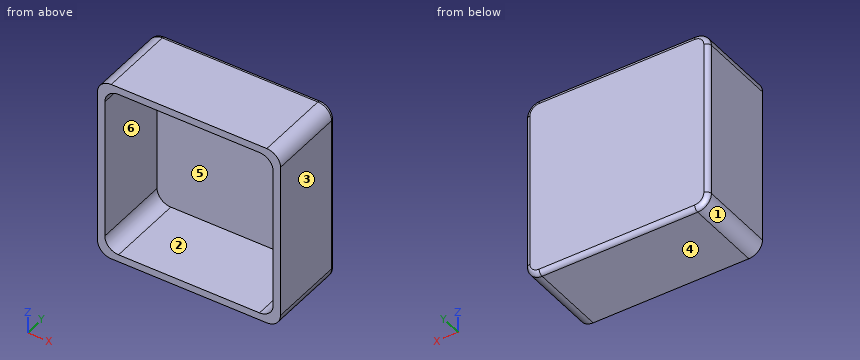
from build123d import *

# Parameters (mm, degrees)
F0_W     = 200
F0_H     = 200
F0_W_2   = 184
F0_H_2   = 184
F1_DEPTH = 85
F2_R     = 15
F4_DEPTH = 3
F5_R     = 5


with BuildPart() as f1:
    # F0 (on Front) → F1 (new body)
    with BuildSketch(Plane.XZ):
        Rectangle(F0_W, F0_H)
        Rectangle(F0_W_2, F0_H_2, mode=Mode.SUBTRACT)
    extrude(amount=F1_DEPTH)

    # F2
    f2_edges = [f1.edges().sort_by_distance(p)[0] for p in [
        (-100, -42.5, 100),
        (-92, -42.5, 92),
        (100, -42.5, 100),
        (92, -42.5, 92),
        (100, -42.5, -100),
        (92, -42.5, -92),
        (-92, -42.5, -92),
        (-100, -42.5, -100),
    ]]
    fillet(f2_edges, radius=F2_R)

    # F3 (on face) → F4 (join)
    with BuildSketch(Plane(origin=(0, 0, 0), x_dir=(-1, 0, 0), z_dir=(0, 1, 0))):
        with BuildLine():
            Line((-85, -100), (85, -100))
            ThreePointArc((85, -100), (95.606602, -95.606602), (100, -85))
            Line((100, -85), (100, 85))
            ThreePointArc((100, 85), (95.606602, 95.606602), (85, 100))
            Line((85, 100), (-85, 100))
            ThreePointArc((-85, 100), (-95.606602, 95.606602), (-100, 85))
            Line((-100, 85), (-100, -85))
            ThreePointArc((-100, -85), (-95.606602, -95.606602), (-85, -100))
        make_face()
    extrude(amount=F4_DEPTH)

    # F5
    f5_edges = [f1.edges().sort_by_distance(p)[0] for p in [
        (95.606602, 3, -95.606602),
    ]]
    fillet(f5_edges, radius=F5_R)


solid = f1.part
The listing builds one solid part. Answer for the finished solid, in the listing's coordinates (mm). Face numbers are marked on the shaded views. A direction names the side the tool comes from. Give positions to 0.01 mm unless a question says otherwise; leave off trailing zeros. Order: outer loops, then holes, each group sorted by start corner. A loop starts at its lowest first (then second) coordinate and runs counter-clockwise, first axis right, second up. Notation, with made-up numbers: (-16.5, 60) - (42.5, 60) arc R7 ccw to (42.5, 67) - close; hole circle Ø7 at (-29.5, 70). An arc over 180 degrees is marked (long way). Answer as CSV lines item,"result".
Q1. Determine the mould class of the marked faces 3, 4, 5 and 6 for opening direction X: pulls with the +X half, pulls with the -X half, needs draft (parallel to the pull), parting line crosses it, or undercut.
Answer key:
face 3,"pulls with the +X half"
face 4,"needs draft"
face 5,"undercut"
face 6,"undercut"
Q2. A cutting plane is placed at C-C, the plane x = 15. Determine the outline of the cut face in (y, z).
Answer key:
outline,"(-85, -100) - (-2, -100) arc R5 ccw to (3, -95) - (3, 95) arc R5 ccw to (-2, 100) - (-85, 100) - (-85, 92) - (0, 92) - (0, -92) - (-85, -92) - close"
Q3. Which of the six approach directions +Z, -Z, +X, -X, +Y, -Y give full straight-line access (tool end or side, diameter ignored) to the marked faces 1 and 2?
Answer key:
face 1,"-Z, -X, +Y, -Y"
face 2,"-Y"
Q4. Straight lines are drawn through the part: L1, parallel to Z at x = -67.5, y = -15; L2, parallel to Y at x = 11, z = -60. For each, find the intervals that lie inside material, in ascending order.
Answer key:
L1,"z = -100 to -92, 92 to 100"
L2,"y = 0 to 3"
Q5. A cutting plane is placed at A-A, the plane y = -15. Determine the outline of the cut face in (x, z).
Answer key:
outline,"(-100, -85) arc R15 ccw to (-85, -100) - (85, -100) arc R15 ccw to (100, -85) - (100, 85) arc R15 ccw to (85, 100) - (-85, 100) arc R15 ccw to (-100, 85) - close; hole (-92, -77) arc R15 ccw to (-77, -92) - (77, -92) arc R15 ccw to (92, -77) - (92, 77) arc R15 ccw to (77, 92) - (-77, 92) arc R15 ccw to (-92, 77) - close"
Q6. This flat-tipped pin is pushed along its axis until it touches: pin 1 Ø6 at (x, z) = (-30.5, -2) entering from -Y. Where does it stop, or does it pass through?
Answer key:
pin 1,"stops at y = 0"
Q7. A cutting plane is placed at B-B, the plane z = -30. Determine the outline of the cut face in (x, y).
Answer key:
outline,"(-100, -85) - (-92, -85) - (-92, 0) - (92, 0) - (92, -85) - (100, -85) - (100, -2) arc R5 ccw to (95, 3) - (-95, 3) arc R5 ccw to (-100, -2) - close"
